Part print with two shaded views. Sizes in mm from the minimum x, y, z corner. Coordinates: 2 decimals unless noted, no trailing zeros. Loops run counter-clockwise (first coordinate to the right, second up) from the corner with the lowest first, then second, coordinate; pieces in that order, holes last.
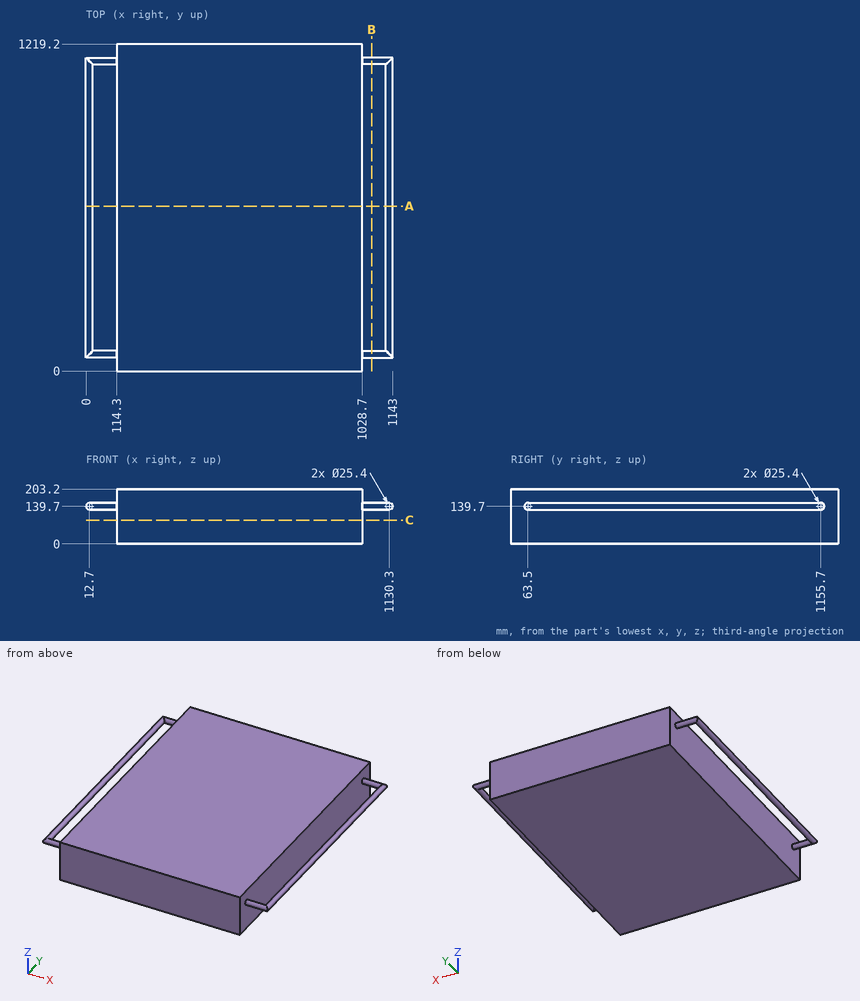
Q1. Slice it at A-A (y = 615). List the corners of the cut face in (x, z).
Answers:
outline: circle Ø25.4 at (12.7, 139.7); (114.3, 0) - (1028.7, 0) - (1028.7, 203.2) - (114.3, 203.2) - close; circle Ø25.4 at (1130.3, 139.7)
Q2. Flat gauge pins, fed straight in: P1, Ø12, axis at y = 971, z = 60, coming from the -X side; P2, Ø5, axis at y = 587.5, z = 127, coming from the +X side. Where does each tip first touch, or does it go through?
Answers:
P1: stops at x = 114.3
P2: stops at x = 1137.87
Q3. Drill centre lines: line 1 (X direction, y = 92.5, z = 139.5); line 2 (X direction, y = 215.5, z = 56); line 3 (X direction, y = 734, z = 133). Where is each one in solid material? Low to high.
Answers:
line 1: x = 0 to 25.4, 114.3 to 1028.7, 1117.6 to 1143
line 2: x = 114.3 to 1028.7
line 3: x = 1.91 to 23.49, 114.3 to 1028.7, 1119.51 to 1141.09
Q4. Slice it at C-C (z = 88.5). List the corners of the cut face in (x, y), and give its area (3 significant figures).
Answers:
outline: (114.3, 0) - (1028.7, 0) - (1028.7, 1219.2) - (114.3, 1219.2) - close
area: 1,110,000 mm2
Q5. Slice it at B-B (x = 1064.5). List the corners of the cut face in (y, z).
Answers:
outline: circle Ø25.4 at (63.5, 139.7); circle Ø25.4 at (1155.7, 139.7)
